from build123d import *

# Parameters (mm, degrees)
CROQUIS1_R              = 17.074936514
SALIENTE_EXTRUIR2_DEPTH = 7
CROQUIS3_R              = 10.273489903
CORTAR_EXTRUIR1_DEPTH   = 4
CROQUIS4_R              = 11.220368527
CORTAR_EXTRUIR2_DEPTH   = 2
CROQUIS5_R              = 10.546758953
CORTAR_EXTRUIR4_DEPTH   = 8
CROQUIS6_R              = 16.523562211
CORTAR_EXTRUIR6_DEPTH   = 6
CROQUIS9_R              = 10.979364786
CROQUIS9_R_2            = 10.546758953
CORTAR_EXTRUIR8_DEPTH   = 1
CROQUIS10_R             = 11.521476728
CROQUIS10_R_2           = 10.979364786
SALIENTE_EXTRUIR3_DEPTH = 1


with BuildPart() as part:
    # Croquis1 → Saliente-Extruir2 (new body)
    with BuildSketch(Plane(origin=(0, 0, 0), x_dir=(1, 0, 0), z_dir=(0, 1, 0))):
        Circle(CROQUIS1_R)
    extrude(amount=SALIENTE_EXTRUIR2_DEPTH)

    # Croquis3 → Cortar-Extruir1 (cut)
    with BuildSketch(Plane(origin=(0, 7, 0), x_dir=(1, 0, 0), z_dir=(0, 1, 0))):
        Circle(CROQUIS3_R)
    extrude(amount=-CORTAR_EXTRUIR1_DEPTH, mode=Mode.SUBTRACT)

    # Croquis4 → Cortar-Extruir2 (cut)
    with BuildSketch(Plane(origin=(0, 0, 0), x_dir=(1, 0, 0), z_dir=(0, 1, 0))):
        Circle(CROQUIS4_R)
    extrude(amount=CORTAR_EXTRUIR2_DEPTH, mode=Mode.SUBTRACT)

    # Croquis5 → Cortar-Extruir4 (cut, through all)
    with BuildSketch(Plane(origin=(0, 0, 0), x_dir=(1, 0, 0), z_dir=(0, 1, 0))):
        Circle(CROQUIS5_R)
    extrude(amount=CORTAR_EXTRUIR4_DEPTH, mode=Mode.SUBTRACT)

    # Croquis6 → Cortar-Extruir6 (cut)
    with BuildSketch(Plane.XZ):
        Circle(CROQUIS6_R)
    extrude(amount=-CORTAR_EXTRUIR6_DEPTH, mode=Mode.SUBTRACT)

    # Croquis9 → Cortar-Extruir8 (cut)
    with BuildSketch(Plane.XZ.offset(-6)):
        Circle(CROQUIS9_R)
        Circle(CROQUIS9_R_2, mode=Mode.SUBTRACT)
    extrude(amount=-CORTAR_EXTRUIR8_DEPTH, mode=Mode.SUBTRACT)

    # Croquis10 → Saliente-Extruir3 (add)
    with BuildSketch(Plane.XZ.offset(-6)):
        Circle(CROQUIS10_R)
        Circle(CROQUIS10_R_2, mode=Mode.SUBTRACT)
    extrude(amount=SALIENTE_EXTRUIR3_DEPTH)


solid = part.part
CAD build for the part. Positions are in the model's coordinates, mm. A direction names the side the tool comes from. Round coordinates to 2 decimals unless told otherwise and drop trailing zeros. Write each loop counter-clockwise with the first axis right and the second up, starting at its lowest first coordinate (ties: lowest second). Pieces come first, ordered by that corner, then holes.
(1) Mould opens along Z. For faces 1 (the face through (-13.55, 3.45, 10.39)), 2 (the face through (-0.24, 7, 11.14)), 3 (the face through (3.4, 6, 11.2)) say: pulls with the +Z half, pulls with the -Z half, needs draft (parallel to the pull), parting line crosses it, or undercut.
(2) Slice it at D-D, the plane z = 13. Write the cut outline in (x, y), and give its area (3 significant figures).
(3) Slice it at A-A, the plane z = 0. Write the cut outline in (x, y), and give its area (3 significant figures).
(4) Drop flat-ended pins along their axis: P1, Ø2, axis at y = 1.5, z = -13, coming from the +X side; P2, Ø18.5, axis at x = 2.5, z = -5, coming from the -Y side; P3, Ø1.5, axis at y = 5, z = -8.5, coming from the -X side. Give the stop position or say it passes through.
(5) Slice it at B-B, the plane x = 0. Write the cut outline in (y, z).
(6) 3-axis set-ups, long thin cutter, end or side, ignore diameter. For faces 4 (the face through (-2.38, 6.01, -10.72)), 5 (the face through (-9.143, 5.507, -7.011)): which of +Z, -Z, +X, -X, +Y, -Y reach the whole face in a straight line?
(7) Probe line 1 along Z through (x, y) = (0, 5.65); line 2 along Z through (x, y) = (0, 6.05); line 3 along Z through (x, y) = (0, 1.4). List the from-to ranges inside material, lowest first.
(8) Slice it at C-C, the plane y = 1.5. Write the cut outline in (x, z), and give its area (3 significant figures).
From the geometry:
1. face 1: parting line crosses it
1. face 2: needs draft
1. face 3: undercut
2. outline: (-11.07, 0) - (-10.2, 0) - (-10.2, 6) - (10.2, 6) - (10.2, 0) - (11.07, 0) - (11.07, 7) - (-11.07, 7) - close
2. area: 32.6 mm2
3. outline: (-17.07, 0) - (-16.52, 0) - (-16.52, 6) - (-11.52, 6) - (-11.52, 5) - (-10.98, 5) - (-10.98, 7) - (-17.07, 7) - close; (10.98, 5) - (11.52, 5) - (11.52, 6) - (16.52, 6) - (16.52, 0) - (17.07, 0) - (17.07, 7) - (10.98, 7) - close
3. area: 19.9 mm2
4. P1: stops at x = 12.15
4. P2: stops at y = 5
4. P3: stops at x = -15.21
5. outline: (0, -17.07) - (7, -17.07) - (7, -10.98) - (5, -10.98) - (5, -11.52) - (6, -11.52) - (6, -16.52) - (0, -16.52) - close; (0, 16.52) - (6, 16.52) - (6, 11.52) - (5, 11.52) - (5, 10.98) - (7, 10.98) - (7, 17.07) - (0, 17.07) - close
6. face 4: +Y, -Y
6. face 5: -Y
7. line 1: z = -17.07 to -16.52, -11.52 to -10.98, 10.98 to 11.52, 16.52 to 17.07
7. line 2: z = -17.07 to -10.98, 10.98 to 17.07
7. line 3: z = -17.07 to -16.52, 16.52 to 17.07
8. outline: circle Ø34.15 at (0, 0); hole circle Ø33.05 at (0, 0)
8. area: 58.2 mm2
